```python
from build123d import *

# Parameters (mm, degrees)
F0_R     = 4.1
F0_R_2   = 1.4
F1_DEPTH = 1.7
F2_R     = 3
F2_R_2   = 1.4
F3_DEPTH = 5
F4_DEPTH = 11.5
F5_R     = 4
F5_R_2   = 1.4
F6_DEPTH = 4


with BuildPart() as f1:
    # F0 (on Top) → F1 (new body)
    with BuildSketch(Plane.XY):
        Circle(F0_R)
        Circle(F0_R_2, mode=Mode.SUBTRACT)
    extrude(amount=-F1_DEPTH)

    # F2 (on face) → F3 (join)
    with BuildSketch(Plane(origin=(0, 0, -1.7), x_dir=(1, 0, 0), z_dir=(0, 0, -1))):
        Circle(F2_R)
        Circle(F2_R_2, mode=Mode.SUBTRACT)
    extrude(amount=F3_DEPTH)

    # F0 (on Top) → F4 (join)
    with BuildSketch(Plane.XY):
        Polygon((5.1961524227, -3), (5.1961524227, 3), (0, 6), (-5.1961524227, 3), (-5.1961524227, -3), (0, -6), align=None)
        Circle(F0_R, mode=Mode.SUBTRACT)
        Circle(F0_R)
        Circle(F0_R_2, mode=Mode.SUBTRACT)
    extrude(amount=F4_DEPTH)

    # F5 (on face) → F6 (join)
    with BuildSketch(Plane.XY.offset(11.5)):
        Circle(F5_R)
        Circle(F5_R_2, mode=Mode.SUBTRACT)
    extrude(amount=F6_DEPTH)


solid = f1.part
```
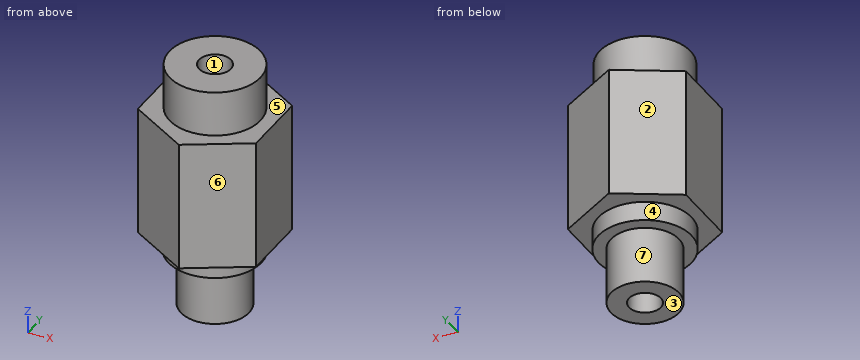
Part model, mm, in its own coordinate system. Face numbers are marked on the shaded views. A direction names the side the tool comes from. Round coordinates to 2 decimals unless told otherwise and drop trailing zeros. Order: outer loops, then holes, each group sorted by start corner. A loop starts at its lowest first (then second) coordinate and runs counter-clockwise, first axis right, second up. Notation, with made-up numbers: M 31.5,37 L 76.5,37 A8 ccw 76.5,41 Z; hole C -37.5,37.5 d8. An arc over 180 degrees is marked long. Put each result on its own line as item: value. Start each with the question number.
1. Drop flat-ended pins along their axis: pin 1 (5 mm diameter, centred on y = -4, z = 5.5, fed in from +X); pin 2 (5 mm diameter, centred on x = 1.5, z = -4, fed in from +Y); pin 3 (1.5 mm diameter, centred on y = -2, z = -2, fed in from -X); pin 4 (1 mm diameter, centred on x = -1, z = 5, fed in from +Y). Give the stop position or say it passes through.
2. Slice it at C-C on x = 0.5. List the corners of the cut face in (y, z), then the cut area to 3 significant figures.
3. Slice it at D-D on z = -5. List the corners of the cut face in (x, y).
4. Drill centre lines: probe 1 along X at (y, z) = (0, 4); probe 2 along Z at (x, y) = (-1.75, -2.75); probe 3 along Y at (x, z) = (-0.25, 1.5). Where is each one in solid material? Low to high. Write a range as [from, to].
5. Two-plate mould, pull along X, no slides. Class the marked faces 1, 2, 3 and 4: +X half, -X half, draft (parallel to the pull), parting line (faces both ways), or undercut.
6. Slice it at B-B on z = 5.5. List the corners of the cut face in (x, y), then the cut area to 3 significant figures.
7. Slice it at A-A on y = 0. List the corners of the cut face in (x, z), then the cut area to 3 significant figures.
8. Tool access for the marked faces 5, 6 and 7: list every direction of +Z, -Z, +X, -X, +Y, -Y with a clear straight run to the whole face (end or side of a thin tool).
Findings:
1. pin 1: x = 5.2
1. pin 2: y = 4.07
1. pin 3: x = -3.88
1. pin 4: y = 5.71
2. outline: M -5.71,0 L -4.07,0 L -4.07,-1.7 L -2.96,-1.7 L -2.96,-6.7 L -1.31,-6.7 L -1.31,15.5 L -3.97,15.5 L -3.97,11.5 L -5.71,11.5 Z; M 1.31,-6.7 L 2.96,-6.7 L 2.96,-1.7 L 4.07,-1.7 L 4.07,0 L 5.71,0 L 5.71,11.5 L 3.97,11.5 L 3.97,15.5 L 1.31,15.5 Z
2. area: 148 mm2
3. outline: C 0,0 d6; hole C 0,0 d2.8
4. probe 1: [-5.2, -1.4], [1.4, 5.2]
4. probe 2: [-1.7, 15.5]
4. probe 3: [-5.86, -1.38], [1.38, 5.86]
5. face 1: undercut
5. face 2: -X half
5. face 3: draft
5. face 4: parting line
6. outline: M -5.2,-3 L 0,-6 L 5.2,-3 L 5.2,3 L 0,6 L -5.2,3 Z; hole C 0,0 d2.8
6. area: 87.4 mm2
7. outline: M -5.2,0 L -4.1,0 L -4.1,-1.7 L -3,-1.7 L -3,-6.7 L -1.4,-6.7 L -1.4,15.5 L -4,15.5 L -4,11.5 L -5.2,11.5 Z; M 1.4,-6.7 L 3,-6.7 L 3,-1.7 L 4.1,-1.7 L 4.1,0 L 5.2,0 L 5.2,11.5 L 4,11.5 L 4,15.5 L 1.4,15.5 Z
7. area: 133 mm2
8. face 5: +Z
8. face 6: +Z, -Z, +X, -Y
8. face 7: -Z
